Read the model definition and answer for the solid it produces. Units are mm, in the model's axes. A direction names the side the tool comes from. Round coordinates to 2 decimals unless told otherwise and drop trailing zeros. Loops run counter-clockwise (first coordinate to the right, second up) from the corner with the lowest first, then second, coordinate; pieces in that order, holes last. Notation, with made-up numbers: (-36.5, 35) -> (-1.5, 35) arc R18 ccw to (-1.5, 43) -> close; hole circle Ø8 at (-26.75, 17). An arc over 180 degrees is marked (long way). Put each result on its own line as item: value.
from build123d import *

# Parameters (mm, degrees)
BOSS_EXTRUDE1_DEPTH = 9.525
SKETCH11_R          = 6.4135
CUT_EXTRUDE7_DEPTH  = 1.5875
SKETCH12_R          = 4.826
CUT_EXTRUDE8_DEPTH  = 23.464106648
SKETCH13_R          = 0.635
CUT_EXTRUDE9_DEPTH  = 25.720183808
FILLET1_R           = 2.54
SKETCH15_W          = 8.472670481
SKETCH15_H          = 13.323689659
SKETCH15_W_2        = 7.661730679
CUT_EXTRUDE10_DEPTH = 28.733584143
FILLET2_R           = 2.54


with BuildPart() as part:
    # Sketch10 → Boss-Extrude1 (new body)
    with BuildSketch(Plane.XY):
        with BuildLine():
            Line((-8.5725, 0), (-8.5725, -4.445))
            Line((-8.5725, -4.445), (-18.7325, -4.445))
            Line((-18.7325, -4.445), (-18.7325, -9.525))
            Line((-18.7325, -9.525), (18.7325, -9.525))
            Line((18.7325, -9.525), (18.7325, -4.445))
            Line((18.7325, -4.445), (8.5725, -4.445))
            Line((8.5725, -4.445), (8.5725, 0))
            ThreePointArc((8.5725, 0), (0, 8.5725), (-8.5725, 0))
        make_face()
    extrude(amount=BOSS_EXTRUDE1_DEPTH)

    # Sketch11 → Cut-Extrude7 (cut)
    with BuildSketch(Plane(origin=(0, 0, 0), x_dir=(-1, 0, 0), z_dir=(0, 0, -1))):
        Circle(SKETCH11_R)
    extrude(amount=-CUT_EXTRUDE7_DEPTH, mode=Mode.SUBTRACT)

    # Sketch12 → Cut-Extrude8 (cut, through all)
    with BuildSketch(Plane(origin=(0, 0, 1.5875), x_dir=(-1, 0, 0), z_dir=(0, 0, -1))):
        Circle(SKETCH12_R)
    extrude(amount=-CUT_EXTRUDE8_DEPTH, mode=Mode.SUBTRACT)

    # Sketch13 → Cut-Extrude9 (cut, through all)
    with BuildSketch(Plane(origin=(0, -4.445, 0), x_dir=(1, 0, 0), z_dir=(0, 1, 0))):
        with Locations(Location((-8.763, -4.7625, 0), (0, 0, 180))):
            Circle(SKETCH13_R)
        with Locations(Location((8.763, -4.7625, 0), (0, 0, 180))):
            Circle(SKETCH13_R)
    extrude(amount=-CUT_EXTRUDE9_DEPTH, mode=Mode.SUBTRACT)

    # Fillet1
    # the kernel refuses this fillet: 2.54 mm, written as the material it adds along each edge
    with BuildSketch(Plane(origin=(8.5725, -4.445, 0), x_dir=(0, 1, 0), z_dir=(0, 0, 1))) as fillet1_piece_1_section:
        with BuildLine():
            CenterArc((FILLET1_R, -FILLET1_R), FILLET1_R, 90, 90)
            Line((0, -FILLET1_R), (0, 0))
            Line((0, 0), (FILLET1_R, 0))
        make_face()
    fillet1_piece_1 = extrude(amount=10.506748607, mode=Mode.PRIVATE)
    fillet1_piece_1 = split(fillet1_piece_1, bisect_by=Plane(origin=(8.63691398, -2.568331275, 9.525), z_dir=(0, 0, -1)), keep=Keep.TOP, mode=Mode.PRIVATE)
    fillet1_piece_1 = fillet1_piece_1 - Plane(origin=(8.763, -2.568331275, 4.7625), x_dir=(-1, 0, 0), z_dir=(0, 1, 0)) * Cylinder(0.635, 32, mode=Mode.PRIVATE)
    add(fillet1_piece_1)
    with BuildSketch(Plane(origin=(-8.5725, -4.445, -0.981748607), x_dir=(0, 1, 0), z_dir=(0, 0, 1))) as fillet1_piece_2_section:
        with BuildLine():
            CenterArc((FILLET1_R, FILLET1_R), FILLET1_R, 180, 90)
            Line((0, FILLET1_R), (0, 0))
            Line((0, 0), (FILLET1_R, 0))
        make_face()
    fillet1_piece_2 = extrude(amount=10.506748607, mode=Mode.PRIVATE)
    fillet1_piece_2 = split(fillet1_piece_2, bisect_by=Plane(origin=(-8.636913982, -2.568331274, 0), z_dir=(0, 0, 1)), keep=Keep.TOP, mode=Mode.PRIVATE)
    fillet1_piece_2 = fillet1_piece_2 - Plane(origin=(-8.763, -2.568331274, 4.7625), x_dir=(-1, 0, 0), z_dir=(0, 1, 0)) * Cylinder(0.635, 32, mode=Mode.PRIVATE)
    add(fillet1_piece_2)
    # the kernel refuses this fillet: 2.54 mm, written as the material it takes off along each edge
    with BuildSketch(Plane(origin=(18.7325, -4.445, -6.35), x_dir=(-1, 0, 0), z_dir=(0, 0, 1)), Plane(origin=(-18.7325, -4.445, -6.35), x_dir=(0, -1, 0), z_dir=(0, 0, 1))) as fillet1_2_piece_1:
        with BuildLine():
            CenterArc((FILLET1_R, FILLET1_R), FILLET1_R, 180, 90)
            Line((0, FILLET1_R), (0, 0))
            Line((0, 0), (FILLET1_R, 0))
        make_face()
    extrude(amount=22.225, mode=Mode.SUBTRACT)

    # Sketch15 → Cut-Extrude10 (cut, through all)
    with BuildSketch(Plane.XZ.offset(9.525)):
        with Locations((-16.809335241, 4.995083112)):
            Rectangle(SKETCH15_W, SKETCH15_H)
        with Locations((16.40386534, 4.995083112)):
            Rectangle(SKETCH15_W_2, SKETCH15_H)
    extrude(amount=-CUT_EXTRUDE10_DEPTH, mode=Mode.SUBTRACT)

    # Fillet2
    fillet2_edges = [part.edges().sort_by_distance(p)[0] for p in [
        (12.573, -4.445, 4.7625),
        (-12.573, -4.445, 4.7625),
    ]]
    fillet(fillet2_edges, radius=FILLET2_R)


solid = part.part
Item 1: For a pull along Y with two mould halves and no side action, classify faces 1 (the cylindrical face through (3.83, -2.937, 5.501)), 2 (the flat face through (3, -4, 9.525)), 3 (the cylindrical face through (-9.72, -4.03, 4.7)) as pulls with the +Y half, pulls with the -Y half, needs draft (parallel to the pull), parting line crosses it, or undercut.
Derived:
face 1: undercut
face 2: needs draft
face 3: pulls with the +Y half
Item 2: The part is cut by section D-D (y = 5.5). Determine the outline of the cut face in (x, z) (1 decimal).
Derived:
outline: (-6.6, 0) -> (-3.3, 0) -> (-3.3, 1.6) -> (3.3, 1.6) -> (3.3, 0) -> (6.6, 0) -> (6.6, 9.5) -> (-6.6, 9.5) -> close
Item 3: The part is cut by section C-C (y = 3.5). Determine the outline of the cut face in (x, z) (1 decimal), then the cut area to 3 significant figures.
Derived:
outline: (-7.8, 0) -> (-5.4, 0) -> (-5.4, 1.6) -> (-3.3, 1.6) -> (-3.3, 9.5) -> (-7.8, 9.5) -> close; (3.3, 1.6) -> (5.4, 1.6) -> (5.4, 0) -> (7.8, 0) -> (7.8, 9.5) -> (3.3, 9.5) -> close
area: 79.3 mm^2
Item 4: The part is cut by section B-B (y = -4). Determine the outline of the cut face in (x, z) (1 decimal).
Derived:
outline: (-9.7, 0) -> (-5, 0) -> (-5, 1.6) -> (-2.7, 1.6) -> (-2.7, 9.5) -> (-9.7, 9.5) -> close; (2.7, 1.6) -> (5, 1.6) -> (5, 0) -> (9.7, 0) -> (9.7, 9.5) -> (2.7, 9.5) -> close; hole (-8.6, 4.2) -> (-8.6, 5.4) arc R0.6 ccw (long way) to start; hole (8.6, 4.2) arc R0.6 ccw (long way) to (8.6, 5.4) -> close
Item 5: Flat-ended cylindrical pins translate along their axes: pin 1 Ø1.3 at (y, z) = (-1.5, 6) entering from -X; pin 2 Ø1.7 at (x, z) = (-8.76, 4.76) entering from +Y; pin 3 Ø3.5 at (y, z) = (-1.5, 2.5) entering from +X. Find the tip coordinate at first contact, or state that the pin passes through.
Derived:
pin 1: stops at x = -8.58
pin 2: stops at y = 3.3
pin 3: stops at x = 8.96
Item 6: The part is cut by section A-A (x = 0). Determine the outline of the cut face in (y, z) (1 decimal), then the cut area to 3 significant figures.
Derived:
outline: (-9.5, 0) -> (-6.4, 0) -> (-6.4, 1.6) -> (-4.8, 1.6) -> (-4.8, 9.5) -> (-9.5, 9.5) -> close; (4.8, 1.6) -> (6.4, 1.6) -> (6.4, 0) -> (8.6, 0) -> (8.6, 9.5) -> (4.8, 9.5) -> close
area: 75.4 mm^2
Item 7: Find the intervals of material crossed by line 1 along Y through (x, z) = (0, 7.25) (1 decimal); line 2 along Y through (x, z) = (0, 0.6) (1 decimal); line 3 along X through (y, z) = (-8, 4.5), in increasing order.
Derived:
line 1: y = -9.5 to -4.8, 4.8 to 8.6
line 2: y = -9.5 to -6.4, 6.4 to 8.6
line 3: x = -12.57 to -9.34, -8.18 to 8.18, 9.34 to 12.57
Item 8: Which of the six approach directions +Z, -Z, +X, -X, +Y, -Y give full straight-line access (tool end or side, diameter ignored) to faces 4 (the flat face through (3, -6, 0)), 5 (the cylindrical face through (9.397, -6.508, 4.79)), 6 (the cylindrical face through (-6.117, 1.926, 0.783))?
Derived:
face 4: -Z, +X, -X, +Y, -Y
face 5: -Y
face 6: -Z
